CAD build for the part. Positions are in the model's coordinates, mm. A direction names the side the tool comes from. Coordinates: 2 decimals unless noted, no trailing zeros. Loops run counter-clockwise (first coordinate to the right, second up) from the corner with the lowest first, then second, coordinate; pieces in that order, holes last.
1) Which spindle directions (+Z, -Z, +X, -X, +Y, -Y) get a long thin tool onto all of the face, cutting with end or side? Do faces 5 (the flat face through (1, -4, -1)), 6 (the flat face through (0, -1, -2)), 7 (the cylindrical face through (-3.486, 0.717, -0.976)). Say none if no direction does.
2) Saw through at A-A, the plane y = -2. Write the cut outline in (x, z), and give its area (3 significant figures).
3) Wall check: line 1 along X through (y, z) = (-1.65, -2.5); line 2 along X through (y, z) = (1.5, -0.5); line 3 along Y through (x, z) = (-0.5, -4). Give the ranges that are in metal, low to high.
4) Saw through at B-B, the plane z = 0. Write the cut outline in (x, y).
5) Saw through at C-C, the plane x = -0.75. Write the cut outline in (y, z), and give its area (3 significant figures).
6) Saw through at D-D, the plane y = 2.5. Write the cut outline in (x, z).
7) Two-plate mould, pull along X, no slides. Class faces 1 (the flat face through (0, -1, 0)), 2 (the flat face through (-2.5, 0.5, -1.2)), 3 (the flat face through (0, -1, 3)), 4 (the flat face through (2.5, 0, 0)): +X half, -X half, draft (parallel to the pull), parting line (faces both ways), or undercut.
```python
from build123d import *

# Parameters (mm, degrees)
F0_W      = 5
F0_H      = 10
F1_DEPTH  = 4
F2_W      = 2
F2_H      = 4
F3_DEPTH  = 25
F4_R      = 2
F7_DEPTH  = 3
F8_DEPTH  = 25
F9_R      = 1
F10_DEPTH = 2


# Not quite as in the source:
# - a feature names something its author has since deleted; it is built from what else it names


with BuildPart() as f1:
    # F0 (on Front) → F1 (new body, symmetric)
    with BuildSketch(Plane.XZ):
        Rectangle(F0_W, F0_H)
    extrude(amount=F1_DEPTH, both=True)

    # F2 (on face) → F3 (cut)
    with BuildSketch(Plane.XZ.offset(4)):
        with Locations((3.5, 3)):
            Rectangle(F2_W, F2_H)
        with Locations((10.5, 3)):
            Rectangle(F2_W, F2_H)
        with Locations((17.5, 3)):
            Rectangle(F2_W, F2_H)
        with Locations((17.5, -3)):
            Rectangle(F2_W, F2_H)
        with Locations((10.5, -3)):
            Rectangle(F2_W, F2_H)
        with Locations((3.5, -3)):
            Rectangle(F2_W, F2_H)
    extrude(amount=-F3_DEPTH, mode=Mode.SUBTRACT)

    # F4
    f4_edges = [f1.edges().sort_by_distance(p)[0] for p in [
        (-2.5, 4, 0),
        (2.5, 4, 0),
    ]]
    fillet(f4_edges, radius=F4_R)

    # F6 (on face) → F7 (cut)
    with BuildSketch(Plane.XZ.offset(4)):
        Polygon((2.5, 5), (0, 5), (-2.5, 5), (-2.5, -5), (2.5, -5), align=None)
        with BuildLine():
            ThreePointArc((2, -2.5), (-1.4142135624, -3.9142135624), (0, -0.5))
            ThreePointArc((0, -0.5), (1.4142135624, -1.0857864376), (2, -2.5))
        make_face(mode=Mode.SUBTRACT)
        with BuildLine():
            ThreePointArc((0, 0.5), (-2, 2.5), (0, 4.5))
            ThreePointArc((0, 4.5), (1.4142135624, 3.9142135624), (2, 2.5))
            ThreePointArc((2, 2.5), (1.4142135624, 1.0857864376), (0, 0.5))
        make_face(mode=Mode.SUBTRACT)
        with BuildLine():
            ThreePointArc((1.5, -2.5), (1.0606601718, -1.4393398282), (0, -1))
            ThreePointArc((0, -1), (-1.0606601718, -3.5606601718), (1.5, -2.5))
        make_face()
        with BuildLine():
            Line((0, 2.5), (0, 4))
            ThreePointArc((0, 4), (-1.5, 2.5), (0, 1))
            Line((0, 1), (0, 2.5))
        make_face()
        with BuildLine():
            ThreePointArc((1.5, 2.5), (1.0606601718, 3.5606601718), (0, 4))
            Line((0, 4), (0, 2.5))
            Line((0, 2.5), (0, 1))
            ThreePointArc((0, 1), (1.0606601718, 1.4393398282), (1.5, 2.5))
        make_face()
    extrude(amount=-F7_DEPTH, mode=Mode.SUBTRACT)

    # F5 (on face) → F8 (cut)
    with BuildSketch(Plane.XY.offset(5)):
        with BuildLine():
            ThreePointArc((2, 1.5), (1.4142135624, 2.9142135624), (0, 3.5))
            ThreePointArc((0, 3.5), (-1.4142135624, 0.0857864376), (2, 1.5))
        make_face()
    extrude(amount=-F8_DEPTH, mode=Mode.SUBTRACT)

    # F9 (on face) → F10 (join)
    with BuildSketch(Plane(origin=(-2.5, 0, 0), x_dir=(0, -1, 0), z_dir=(-1, 0, 0))):
        with Locations((-0.5, 0)):
            Circle(F9_R)
    extrude(amount=F10_DEPTH)


solid = f1.part
```
Data:
1. face 5: +Z, -Z, +X, -X, -Y
1. face 6: -Y
1. face 7: -X
2. outline: circle Ø4 at (0, -2.5); circle Ø4 at (0, 2.5); hole circle Ø3 at (0, -2.5); hole circle Ø3 at (0, 2.5)
2. area: 11.0 mm2
3. line 1: x = -2 to -1.5, 1.5 to 2
3. line 2: x = -2.5 to -2, 2 to 2.5
3. line 3: y = -4 to -0.44, 3.44 to 4
4. outline: (-4.5, -0.5) - (-2.5, -0.5) - (-2.5, -1) - (2.5, -1) - (2.5, 2) arc R2 ccw to (0.5, 4) - (-0.5, 4) arc R2 ccw to (-2.5, 2) - (-2.5, 1.5) - (-4.5, 1.5) - close; hole circle Ø4 at (0, 1.5)
5. outline: (-4, -4.35) - (-1, -4.35) - (-1, -5) - (-0.35, -5) - (-0.35, 5) - (-1, 5) - (-1, 4.35) - (-4, 4.35) - (-4, 3.8) - (-1, 3.8) - (-1, 1.2) - (-4, 1.2) - (-4, 0.65) - (-1, 0.65) - (-1, -0.65) - (-4, -0.65) - (-4, -1.2) - (-1, -1.2) - (-1, -3.8) - (-4, -3.8) - close; (3.35, -5) - (3.98, -5) - (3.98, 5) - (3.35, 5) - close
5. area: 19.4 mm2
6. outline: (-2.44, -5) - (-1.73, -5) - (-1.73, 5) - (-2.44, 5) - close; (1.73, -5) - (2.44, -5) - (2.44, 5) - (1.73, 5) - close
7. face 1: draft
7. face 2: -X half
7. face 3: undercut
7. face 4: +X half
